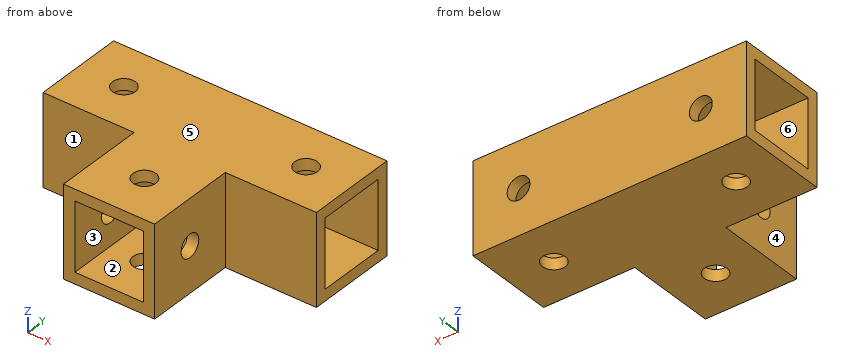
```python
from build123d import *

# Parameters (mm, degrees)
F1_DEPTH = 20
F2_T     = -2.5
F3_R     = 2.5
F4_DEPTH = 20.001
F5_R     = 2.5
F6_DEPTH = 2.5
F7_R     = 2.5
F8_DEPTH = 40.001


with BuildPart() as f1:
    # F0 (on Top) → F1 (new body)
    with BuildSketch(Plane.XY):
        Polygon((30, 0), (-30, 0), (-30, -20), (-10, -20), (-10, -40), (10, -40), (10, -20), (30, -20), align=None)
    extrude(amount=-F1_DEPTH)

    # F2
    f2_openings = [f1.faces().sort_by_distance(p)[0] for p in [
        (30, -10, -10),
        (0, -40, -10),
        (-30, -10, -10),
    ]]
    offset(amount=F2_T, openings=f2_openings, kind=Kind.INTERSECTION)

    # F3 (on face) → F4 (cut, through all)
    with BuildSketch(Plane.XY):
        with Locations((-20, -10)):
            Circle(F3_R)
        with Locations((20, -10)):
            Circle(F3_R)
        with Locations((0, -30)):
            Circle(F3_R)
    extrude(amount=-F4_DEPTH, mode=Mode.SUBTRACT)

    # F5 (on face) → F6 (cut, through all)
    with BuildSketch(Plane(origin=(0, 0, 0), x_dir=(-1, 0, 0), z_dir=(0, 1, 0))):
        with Locations((-20, -10)):
            Circle(F5_R)
        with Locations((20, -10)):
            Circle(F5_R)
    extrude(amount=-F6_DEPTH, mode=Mode.SUBTRACT)

    # F7 (on face) → F8 (cut, through all)
    with BuildSketch(Plane.YZ.offset(10)):
        with Locations((-30, -10)):
            Circle(F7_R)
    extrude(amount=-F8_DEPTH, mode=Mode.SUBTRACT)


solid = f1.part
```
For this review, take the finished solid that the model builds, in its own axes (mm). Face numbers are marked on the shaded views. A direction names the side the tool comes from. Round coordinates to 2 decimals unless told otherwise and drop trailing zeros. Write each loop counter-clockwise with the first axis right and the second up, starting at its lowest first coordinate (ties: lowest second). Pieces come first, ordered by that corner, then holes. Notation, with made-up numbers: (57.5, 21) - (81.5, 21) arc R33 ccw to (81.5, 49) - close; hole circle Ø10 at (-0.5, 51). An arc over 180 degrees is marked (long way). Write each question's results on one line, items separated by ' | '.
Item 1: For the marked faces 1, 2 and 3, list the 3-axis set-ups (+Z, -Z, +X, -X, +Y, -Y) from which the entire face can be reached by the end or side of a thin tool; tool diameter is ignored.
Calculated:
face 1: +Z, -Z, -X, -Y | face 2: none | face 3: -Y
Item 2: Take a section at A-A on y = -10. State the section outline as (x, z) points.
Calculated:
outline: (-30, -20) - (-22.5, -20) - (-22.5, -17.5) - (-30, -17.5) - close; (-30, -2.5) - (-22.5, -2.5) - (-22.5, 0) - (-30, 0) - close; (-17.5, -20) - (17.5, -20) - (17.5, -17.5) - (-17.5, -17.5) - close; (-17.5, -2.5) - (17.5, -2.5) - (17.5, 0) - (-17.5, 0) - close; (22.5, -20) - (30, -20) - (30, -17.5) - (22.5, -17.5) - close; (22.5, -2.5) - (30, -2.5) - (30, 0) - (22.5, 0) - close
Item 3: To check wall thickness, follow line 1 along Y through (x, z) = (17, -4); line 2 along Y through (x, z) = (0, -1.05). State the ranges of each line that lie inside material, in increasing order. Write a range as from..to.
Calculated:
line 1: y = -20..-17.5, -2.5..0 | line 2: y = -40..-32.5, -27.5..0
Item 4: For pin 1 (7.5 mm diameter, centred on y = -32.5, z = -7, fed in from +X); pin 2 (7.5 mm diameter, centred on y = -29.5, z = -10, fed in from -X); pin 3 (6 mm diameter, centred on x = 20, z = -6.5, fed in from -Y), all flat-tipped, find the tip position at first contact; note any pin that passes through.
Calculated:
pin 1: stops at x = 10 | pin 2: stops at x = -10 | pin 3: stops at y = -20
Item 5: Take a section at C-C on x = 0. State the section outline as (y, z) points.
Calculated:
outline: (-40, -20) - (-32.5, -20) - (-32.5, -17.5) - (-40, -17.5) - close; (-40, -2.5) - (-32.5, -2.5) - (-32.5, 0) - (-40, 0) - close; (-27.5, -20) - (0, -20) - (0, 0) - (-27.5, 0) - (-27.5, -2.5) - (-2.5, -2.5) - (-2.5, -17.5) - (-27.5, -17.5) - close
Item 6: Draft analysis for pull direction Z (two halves, no side actions). For the marked faces 4, 5 and 6, state which applies: pulls with the +Z half, pulls with the -Z half, needs draft (parallel to the pull), parting line crosses it, or undercut.
Calculated:
face 4: needs draft | face 5: pulls with the +Z half | face 6: undercut
Item 7: Take a section at B-B on z = -10. Count the separate pieces of the cut face and the enclosed holes in it, then the cut area to 4 significant figures.
Calculated:
separate pieces: 7 | enclosed holes: 0 | area: 312.5 mm^2
Item 8: Take a section at D-D on y = -31.5. State the section outline as (x, z) points, then the cut area to 3 significant figures.
Calculated:
outline: (-10, -20) - (-2, -20) - (-2, -17.5) - (-7.5, -17.5) - (-7.5, -12) - (-10, -12) - close; (-10, -8) - (-7.5, -8) - (-7.5, -2.5) - (-2, -2.5) - (-2, 0) - (-10, 0) - close; (2, -20) - (10, -20) - (10, -12) - (7.5, -12) - (7.5, -17.5) - (2, -17.5) - close; (2, -2.5) - (7.5, -2.5) - (7.5, -8) - (10, -8) - (10, 0) - (2, 0) - close | area: 135 mm^2
